Could you check a few things on this drawing? It's one solid part, dimensions in mm from its lowest x, y, z. Coordinates: 2 decimals unless noted, no trailing zeros. Write each loop counter-clockwise with the first axis right and the second up, starting at its lowest first coordinate (ties: lowest second). Pieces come first, ordered by that corner, then holes.
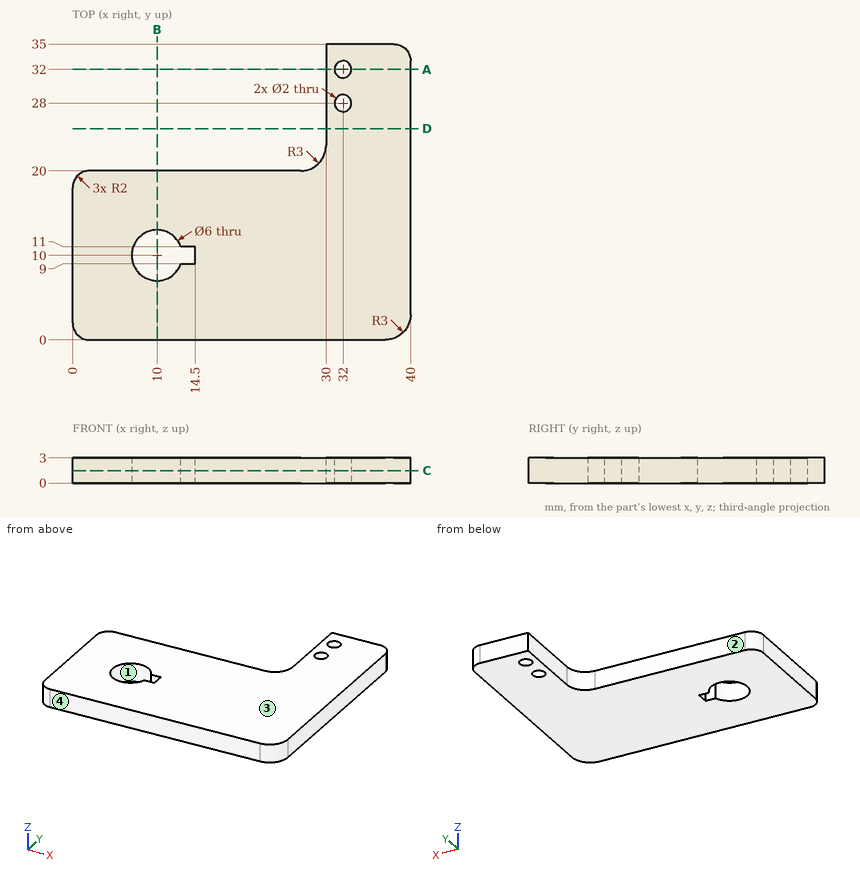
1) Imagine slicing it at D-D on y = 25. Please give me the cut outline in (x, z).
Values follow:
outline: (30, 0) - (40, 0) - (40, 3) - (30, 3) - close
2) We'd pull the mould along Y, two halves only. Please class the marked faces 1, 2, 3 and 4: pulls with the +Y half, pulls with the -Y half, needs draft (parallel to the pull), parting line crosses it, or undercut.
Values follow:
face 1: undercut
face 2: pulls with the +Y half
face 3: needs draft
face 4: pulls with the -Y half
3) Will these pins go through, and if not, where does the flat tip stop? pin 1 (1.8 mm diameter, centred on x = 32, y = 32, fed in from +Z); pin 2 (1.3 mm diameter, centred on x = 14, z = 1.5, fed in from +Y).
Values follow:
pin 1: passes through
pin 2: stops at y = 20
4) I need wall thicknesses on probe 1 along Y at (x, z) = (32, 2.1); probe 2 along X at (y, z) = (10, 1.6); probe 3 along Y at (x, z) = (10, 1.1). Which ranges of each line are inside material? Lowest first, please.
Values follow:
probe 1: y = 0 to 27, 29 to 31, 33 to 35
probe 2: x = 0 to 7, 14.5 to 40
probe 3: y = 0 to 7, 13 to 20
5) Imagine slicing it at A-A on y = 32. Please give me the cut outline in (x, z).
Values follow:
outline: (30, 0) - (31, 0) - (31, 3) - (30, 3) - close; (33, 0) - (40, 0) - (40, 3) - (33, 3) - close
6) Imagine slicing it at C-C on z = 1.5. Please give me the cut outline in (x, y).
Values follow:
outline: (0, 2) arc R2 ccw to (2, 0) - (37, 0) arc R3 ccw to (40, 3) - (40, 33) arc R2 ccw to (38, 35) - (30, 35) - (30, 23) arc R3 cw to (27, 20) - (2, 20) arc R2 ccw to (0, 18) - close; hole (12.83, 9) - (14.5, 9) - (14.5, 11) - (12.83, 11) arc R3 ccw (long way) to start; hole circle Ø2 at (32, 28); hole circle Ø2 at (32, 32)
7) Imagine slicing it at B-B on x = 10. Please give me the cut outline in (y, z), then the cut area to 3 significant figures.
Values follow:
outline: (0, 0) - (7, 0) - (7, 3) - (0, 3) - close; (13, 0) - (20, 0) - (20, 3) - (13, 3) - close
area: 42.0 mm2
